Source: CAD feature listing. Evaluate the final solid. Frame: model axes, mm. Coordinates: 2 decimals unless noted, no trailing zeros. Order: outer loops, then holes, each group sorted by start corner. A loop starts at its lowest first (then second) coordinate and runs counter-clockwise, first axis right, second up.
Autodesk Inventor part; units mm, degrees
ref_plane "YZ Plane" through (0, 0, 0) normal (1, 0, 0) x (0, 1, 0)
ref_plane "XZ Plane" through (0, 0, 0) normal (0, 1, 0) x (-1, 0, 0)
ref_plane "XY Plane" through (0, 0, 0) normal (0, 0, 1) x (1, 0, 0)
sketch "Sketch1" plane through (0, 0, 0) normal (0, 0, 1) x (1, 0, 0)
  circle A0 centre (0, 0) radius 25.4
  line L0 (0, 25.4) -> (-203.2, 25.4)
  line L1 (-203.2, 25.4) -> (-203.2, -12.7)
  line L2 (25.4, 0) -> (203.2, 0) construction
  line L3 (203.2, 0) -> (203.2, -127) construction
  arc A1 (203.2, -127) -> (-203.2, -12.7) centre (-98.0265, -418.3887) ccw construction
  line L4 (-203.2, 25.4) -> (-203.2, -50.8) construction
  arc A2 (203.2, -222.1538) -> (-203.2, -12.7) centre (-125.6377, -361.1999) ccw
  line L5 (-203.2, 25.4) -> (-203.2, 36.3602)
  line L6 (25.4, 0) -> (25.4, 25.4)
  line L7 (25.4, 25.4) -> (0, 25.4)
  circle A3 centre (0, 549.5888) radius 46.99
  line L8 (0, 596.5788) -> (-190.5, 596.5788)
  line L9 (46.99, 549.5888) -> (46.99, 596.5788)
  line L10 (46.99, 596.5788) -> (0, 596.5788)
  line L11 (46.99, 596.5788) -> (224.79, 596.5788)
  line L12 (224.79, 596.5788) -> (224.79, 190.1788)
  line L13 (0, 596.5788) -> (-190.5, 596.5788) construction
  line L14 (-190.5, 596.5788) -> (-190.5, 558.4788) construction
  line L15 (-190.5, 596.5788) -> (-190.5, 558.4788)
  line L16 (-190.5, 596.5788) -> (0, 596.5788)
  line L17 (0, 596.5788) -> (-101.6, 596.5788)
  line L18 (-101.6, 596.5788) -> (-101.6, 545.7788)
  line L19 (-101.6, 545.7788) -> (-46.99, 545.7788)
  line L20 (224.79, 190.1788) -> (-334.01, 190.1788)
  line L21 (23.495, -36.812) -> (-174.1484, -525.1707)
  line L22 (203.2, -222.1538) -> (-203.2, -12.7)
  line L23 (224.79, 264.9183) -> (-394.0921, 264.9183)
  line L24 (224.79, 596.5788) -> (224.79, 393.3788)
  line L25 (224.79, 393.3788) -> (-334.01, 393.3788)
  line L26 (0, 502.5988) -> (0, 393.3788)
  arc A4 (-101.6, 545.7788) -> (-247.5257, 560.3429) centre (-190.5, 393.3788) ccw
  spline S0 degree 2 poles (-101.6, 545.7788) (2.3295, 495.7011) (-25.4, 510.0552) knots 0 0 0 1 1 1
  point P0 (-19.5605, 506.8635)
  point P1 (-190.5, 569.8128)
  dimension "d0" = 50.8
  dimension "d1" = 203.2
  dimension "d2" = 177.8
  dimension "d3" = 127
  dimension "d4" = 38.1
  dimension "d5" = 419.1
  dimension "d6" = 76.2
  dimension "d7" = 457.2
  dimension "d8" = 93.98
  dimension "d11" = 177.8
  dimension "d12" = 406.4
  dimension "d13" = 190.5
  dimension "d14" = 38.1
  dimension "d18" = 101.6
  dimension "d19" = 558.8
  dimension "d20" = 203.2
  dimension "d21" = 558.8
extrude "Extrusion2" add sketch "Sketch1" along normal blind 1.5875 contours A3 S0 | A3 L10 L9 | A3 S0 L18 L8 | S0 A3 | L18 A4 L15 L8
fillet "Fillet2" radius 28.575 1 edges at (46.99, 596.5788, 0.7937)
fillet "Fillet3" radius 3.175 1 edges at (-190.5, 596.5788, 0.7937)
fillet "Fillet4" radius 3.175 1 edges at (-190.5, 569.8128, 0.7937)
sketch "Sketch3" plane through (0, 0, 1.5875) normal (0, 0, 1) x (1, 0, 0)
  circle A0 centre (-186.1685, 576.5475) radius 2.54
  point P0 (0, 0)
  dimension "d27" = 5.08
sketch "Sketch4" plane through (0, 0, 1.5875) normal (0, 0, 1) x (1, 0, 0)
  line L0 (-190.5, 593.4038) -> (-190.5, 572.9597)
  line L1 (46.99, 549.5888) -> (46.99, 568.0038)
  point P0 (0, 0)
properties part number "Better intake poly"
Q1. Material intervals for line 1 along Y through (x, z) = (-125.5, 1.3); line 2 along Y through (x, z) = (-8.5, 0.9); line 3 along X through (y, z) = (511, 1.2), sorted ascending.
Solutions:
line 1: y = 557.4 to 596.58
line 2: y = 503.37 to 596.58
line 3: x = -28.86 to 26.81
Q2. Section query A-A on x = -172. Output: boundary loops of the cut face in (y, z).
Solutions:
outline: (568.84, 0) - (596.58, 0) - (596.58, 1.59) - (568.84, 1.59) - close
Q3. Pin query (flat end, axial travel): P1, Ø8, axis at x = -44, y = 576, coming from the -Z side. Return the tip coordinate at first contact, or that it passes through.
Solutions:
P1: stops at z = 0
Q4. Section query B-B on y = 564. Output: boundary loops of the cut face in (x, z).
Solutions:
outline: (-145.58, 0) - (46.99, 0) - (46.99, 1.59) - (-145.58, 1.59) - close
